Answer from the drawing. Dimensions are ordinates in mm from the lowest x, y and z of the part. A direction names the side the tool comes from. Give positions to 0.01 mm unless a question says otherwise; leave off trailing zeros. Loops run counter-clockwise (first coordinate to the right, second up) from the corner with the lowest first, then second, coordinate; pieces in that order, holes last. Notation, with made-up numbers: (49, -6) - (84, -6) arc R14 ccw to (84, 3) - close; hole circle Ø10 at (-30.5, -3). An arc over 180 degrees is marked (long way). Answer as CSV lines item,"result". Start each with the question number.
1) Flat-ended cylindrical pins translate along their axes: pin 1 (8 mm diameter, centred on y = 13.5, z = 11, fed in from -X); pin 2 (6 mm diameter, centred on x = 23.5, y = 11, fed in from -Z); pin 3 (4 mm diameter, centred on y = 28.5, z = 12, fed in from -X); pin 4 (8 mm diameter, centred on y = 32.5, z = 6.5, fed in from -X). Find the tip coordinate at first contact, or state that the pin passes through.
2) A cutting plane is placed at D-D (z = 8.25). Determine the outline of the cut face in (x, y), and give its area (3 significant figures).
3) A cutting plane is placed at B-B (z = 3.25). Determine the outline of the cut face in (x, y) (1 decimal), and give its area (3 significant figures).
4) Find the intervals of material crossed by line 1 along Y through (x, z) = (15.5, 7) (1 decimal); line 2 along X through (y, z) = (9.5, 2.75) (1 decimal); line 3 along Y through (x, z) = (31, 1.5) (1 decimal), in increasing order.
5) For the marked faces 1, 2 and 3, determine the directions among +Z, -Z, +X, -X, +Y, -Y from which every point of the face is accessible in a straight line to the end or side of a thin tool.
6) A cutting plane is placed at C-C (x = 26.5). Determine the outline of the cut face in (y, z) (1 decimal).
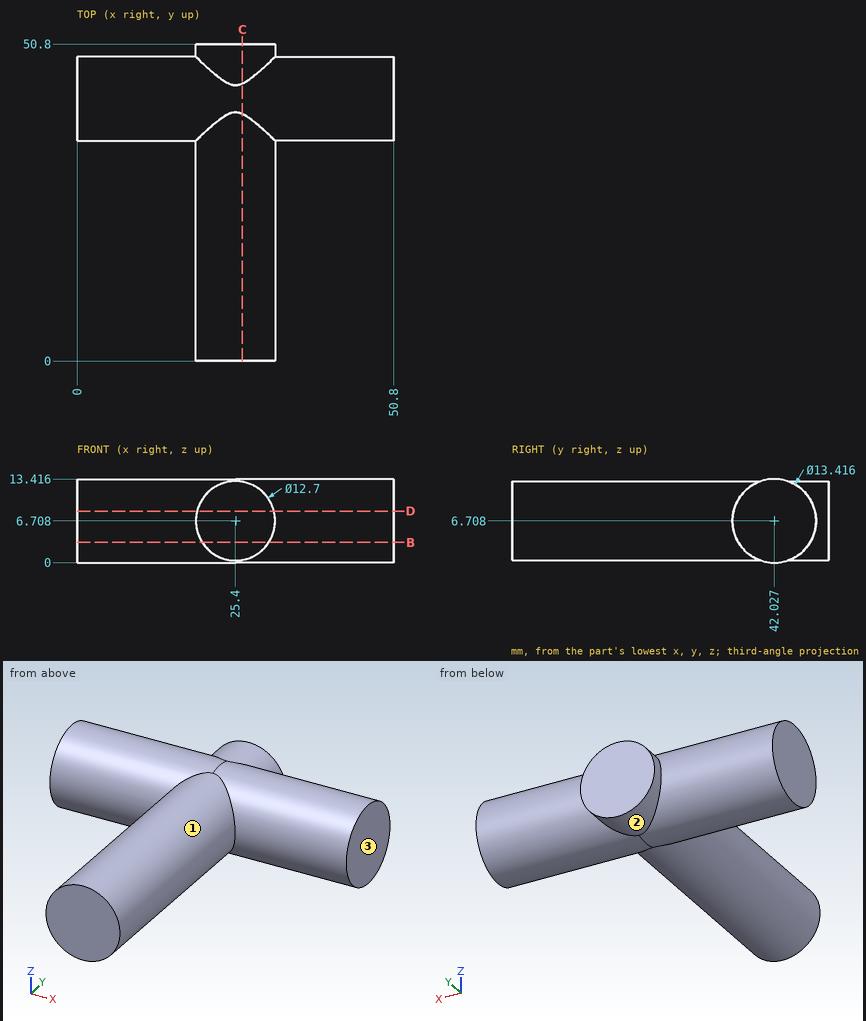
Ans:
1,pin 1,"x = 19.06"
1,pin 2,"z = 0.36"
1,pin 3,"x = 19.97"
1,pin 4,"x = 0"
2,outline,"(0, 35.5) - (19.24, 35.5) - (19.24, 0) - (31.56, 0) - (31.56, 35.5) - (50.8, 35.5) - (50.8, 48.56) - (31.56, 48.56) - (31.56, 50.8) - (19.24, 50.8) - (19.24, 48.56) - (0, 48.56) - close"
2,area,"1,130 mm2"
3,outline,"(0, 36.3) - (20.1, 36.3) - (20.1, 0) - (30.7, 0) - (30.7, 36.3) - (50.8, 36.3) - (50.8, 47.8) - (30.7, 47.8) - (30.7, 50.8) - (20.1, 50.8) - (20.1, 47.8) - (0, 47.8) - close"
3,area,"1,000 mm2"
4,line 1,"35.3 to 48.7"
4,line 2,"20.4 to 30.4"
4,line 3,"37.8 to 46.3"
5,face 1,"-Y"
5,face 2,"+Y"
5,face 3,"+Z, -Z, +X, +Y, -Y"
6,outline,"(0, 0.5) - (39.6, 0.5) arc R6.7 ccw to (44.5, 0.5) - (50.8, 0.5) - (50.8, 13) - (44.5, 13) arc R6.7 ccw to (39.6, 13) - (0, 13) - close"
